Could you check a few things on this model? Use its own coordinates, in mm. Give positions to 0.01 mm unless a question says otherwise; leave off trailing zeros. Write each loop counter-clockwise with the first axis right and the second up, starting at its lowest first coordinate (ties: lowest second). Pieces come first, ordered by that corner, then holes. Notation, with made-up numbers: (67.25, 36) - (126.25, 36) arc R19 cw to (126.25, 69) - close; hole circle Ø4 at (17, 19.25). An arc over 180 degrees is marked (long way). Answer as CSV lines item,"result". Start each with the question number.
Q1. Will these pins go through, and if not, where does the flat tip stop? pin 1 Ø3 at (x, y) = (39.5, -42.5) entering from -Z; pin 2 Ø1.9 at (x, y) = (-36.2, 42.85) entering from +Z.
Q2. If I drill on line 1 along X through (y, z) = (-42.85, 0.3); line 2 along X through (y, z) = (42.85, 0.2); line 3 along Y through (x, z) = (-40, 1.25), over which ranges is the centre line in solid material (lowest first)?
Q3. Imagine slicing it at A-A on y = 42.85. List the corners of the cut face in (x, z) for me.
```python
from build123d import *

# Parameters (mm, degrees)
F0_W           = 90.2
F0_H           = 95.9
F1_DEPTH       = 1.6
F2_D           = 3.2
F2_CBORE_D     = 6.4
F2_CBORE_DEPTH = 0.5
F3_D           = 3.2
F3_CBORE_D     = 6.4
F3_CBORE_DEPTH = 0.5
F4_D           = 3.2
F4_CBORE_D     = 6.4
F4_CBORE_DEPTH = 0.5
F5_D           = 3.2
F5_CBORE_D     = 6.4
F5_CBORE_DEPTH = 0.5


with BuildPart() as f1:
    # F0 (on Top) → F1 (new body)
    with BuildSketch(Plane.XY):
        Rectangle(F0_W, F0_H)
    extrude(amount=F1_DEPTH)

    # F2 (through all)
    with Locations(Plane(origin=(0, 0, 0), x_dir=(1, 0, 0), z_dir=(0, 0, -1))):
        with Locations((-36.2, -42.85)):
            CounterBoreHole(F2_D / 2, F2_CBORE_D / 2, F2_CBORE_DEPTH)

    # F3 (through all)
    with Locations(Plane(origin=(0, 0, 0), x_dir=(1, 0, 0), z_dir=(0, 0, -1))):
        with Locations((-40, 42.85)):
            CounterBoreHole(F3_D / 2, F3_CBORE_D / 2, F3_CBORE_DEPTH)

    # F4 (through all)
    with Locations(Plane(origin=(0, 0, 0), x_dir=(1, 0, 0), z_dir=(0, 0, -1))):
        with Locations((36.2, -42.85)):
            CounterBoreHole(F4_D / 2, F4_CBORE_D / 2, F4_CBORE_DEPTH)

    # F5 (through all)
    with Locations(Plane(origin=(0, 0, 0), x_dir=(1, 0, 0), z_dir=(0, 0, -1))):
        with Locations((40, 42.85)):
            CounterBoreHole(F5_D / 2, F5_CBORE_D / 2, F5_CBORE_DEPTH)


solid = f1.part
```
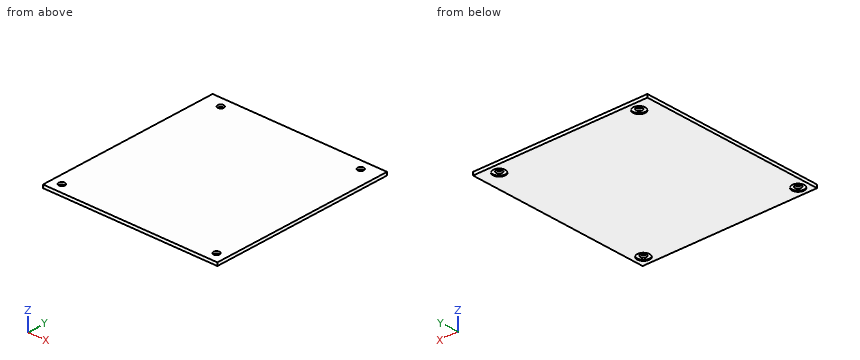
Conclusion:
1,pin 1,"z = 0.5"
1,pin 2,"through"
2,line 1,"-45.1 to -43.2, -36.8 to 36.8, 43.2 to 45.1"
2,line 2,"-45.1 to -39.4, -33 to 33, 39.4 to 45.1"
2,line 3,"-47.95 to -44.45, -41.25 to 47.95"
3,outline,"(-45.1, 0) - (-39.4, 0) - (-39.4, 0.5) - (-37.8, 0.5) - (-37.8, 1.6) - (-45.1, 1.6) - close; (-34.6, 0.5) - (-33, 0.5) - (-33, 0) - (33, 0) - (33, 0.5) - (34.6, 0.5) - (34.6, 1.6) - (-34.6, 1.6) - close; (37.8, 0.5) - (39.4, 0.5) - (39.4, 0) - (45.1, 0) - (45.1, 1.6) - (37.8, 1.6) - close"
